```python
from build123d import *

# Parameters (mm, degrees)
F_9_64_0_14063_DIAMETER_HOLE2_D           = 3.572002
F_9_64_0_14063_DIAMETER_HOLE2_CSINK_D     = 4.842002
F_9_64_0_14063_DIAMETER_HOLE2_CSINK_ANGLE = 100
F_9_64_0_14063_DIAMETER_HOLE3_D           = 3.572002
F_9_64_0_14063_DIAMETER_HOLE3_CSINK_D     = 4.842002
F_9_64_0_14063_DIAMETER_HOLE3_CSINK_ANGLE = 100
CUT_EXTRUDE1_DEPTH                        = 3.81


with BuildPart() as part:
    # Sketch2 → Revolve1 (revolve)
    with BuildSketch(Plane.XY, mode=Mode.PRIVATE) as revolve1_sk:
        with BuildLine():
            Line((0, 0), (-35.56, 0))
            ThreePointArc((-35.56, 0), (-34.441376421, 45.516946226), (-48.26, 88.9))
            Line((-48.26, 88.9), (-50.8, 88.9))
            ThreePointArc((-50.8, 88.9), (-36.890578114, 45.529917412), (-38.1, 0))
            Line((-38.1, 0), (-38.1, -7.62))
            Line((-38.1, -7.62), (0, -7.62))
            Line((0, -7.62), (0, 0))
        make_face()
    revolve(revolve1_sk.sketch.rotate(Axis((0, 0, 0), (0, 1, 0)), 270), axis=Axis((0, 0, 0), (0, 1, 0)))

    # 9/64 (0.14063) Diameter Hole2 (through all)
    with Locations(Plane(origin=(0, 0, 0), x_dir=(1, 0, 0), z_dir=(0, 1, 0))):
        with Locations((0, -28.72641934), (-28.389650063, 0), (0, 28.72641934), (28.120234641, 0), (17.815094761, -20.105125845), (17.815094761, 19.431587291), (-18.421279459, 19.431587291), (-18.421279459, -20.105125845), (0, 0)):
            CounterSinkHole(F_9_64_0_14063_DIAMETER_HOLE2_D / 2, F_9_64_0_14063_DIAMETER_HOLE2_CSINK_D / 2, counter_sink_angle=F_9_64_0_14063_DIAMETER_HOLE2_CSINK_ANGLE)

    # 9/64 (0.14063) Diameter Hole3 (through all)
    with Locations(Plane(origin=(0, -7.62, 0), x_dir=(-1, 0, 0), z_dir=(0, -1, 0))):
        with Locations((-6.364939338, 18.960110303), (7.50995488, 18.960110303), (19.835710423, 7.914078013), (-19.29687958, 7.914078013), (-19.29687958, -8.385555001), (-7.038477892, -21.317495243), (7.914078013, -21.317495243), (19.835710423, -8.857031989)):
            CounterSinkHole(F_9_64_0_14063_DIAMETER_HOLE3_D / 2, F_9_64_0_14063_DIAMETER_HOLE3_CSINK_D / 2, counter_sink_angle=F_9_64_0_14063_DIAMETER_HOLE3_CSINK_ANGLE)

    # Sketch11 → Cut-Extrude1 (cut)
    with BuildSketch(Plane.XZ.offset(7.62)):
        with BuildLine():
            Line((-4.696611831, 37.809414665), (-4.696611831, 30.726938113))
            ThreePointArc((-4.696611831, 30.726938113), (-21.519829113, 22.429887281), (-30.506179441, 5.964554001))
            Line((-30.506179441, 5.964554001), (-37.630228482, 5.964554001))
            ThreePointArc((-37.630228482, 5.964554001), (-38.099253822, 0.238449554), (-37.701937681, -5.493077013))
            Line((-37.701937681, -5.493077013), (-30.594590918, -5.493077013))
            ThreePointArc((-30.594590918, -5.493077013), (-21.692260933, -22.263169229), (-4.696611831, -30.726938113))
            Line((-4.696611831, -30.726938113), (-4.696611831, -37.809414665))
            ThreePointArc((-4.696611831, -37.809414665), (0, -38.1), (4.696611831, -37.809414665))
            Line((4.696611831, -37.809414665), (4.696611831, -30.726938113))
            ThreePointArc((4.696611831, -30.726938113), (21.692260933, -22.263169229), (30.594590918, -5.493077013))
            Line((30.594590918, -5.493077013), (37.701937681, -5.493077013))
            ThreePointArc((37.701937681, -5.493077013), (38.099253822, 0.238449554), (37.630228482, 5.964554001))
            Line((37.630228482, 5.964554001), (30.506179441, 5.964554001))
            ThreePointArc((30.506179441, 5.964554001), (21.519829113, 22.429887281), (4.696611831, 30.726938113))
            Line((4.696611831, 30.726938113), (4.696611831, 37.809414665))
            ThreePointArc((4.696611831, 37.809414665), (0, 38.1), (-4.696611831, 37.809414665))
        make_face()
    extrude(amount=-CUT_EXTRUDE1_DEPTH, mode=Mode.SUBTRACT)


solid = part.part
```
Here's how the part is built. I have some questions about the finished solid (model axes, mm). A direction names the side the tool comes from. Round coordinates to 2 decimals unless told otherwise and drop trailing zeros. Loops run counter-clockwise (first coordinate to the right, second up) from the corner with the lowest first, then second, coordinate; pieces in that order, holes last.
1. Thinking about a two-plate mould opening in X: for faces 1 (the face through (0.387, -2.194, -26.983)), 2 (the face through (-34, -6, -5.493)), 3 (the face through (14.593, -3.863, -35.195)), which applies, released by +X, released by -X, zero draft, split by the parting line, or undercut?
Answers:
face 1: undercut
face 2: zero draft
face 3: split by the parting line
2. If I drill on probe 1 along Z at (x, y) = (5, 19); probe 2 along X at (y, z) = (57, 4); probe 3 along Z at (x, y) = (10.5, 61), over which ranges is the centre line in solid material (lowest first)?
Answers:
probe 1: z = -35.37 to -32.87, 32.87 to 35.37
probe 2: x = -38.83 to -36.36, 36.36 to 38.83
probe 3: z = -38.63 to -36.07, 36.07 to 38.63
3. Suppose I cut it at D-D, the plane y = 20.5. Please give me the cut outline in (x, z).
Answers:
outline: circle Ø71.3 at (0, 0); hole circle Ø66.35 at (0, 0)
4. Suppose I cut it at A-A, the plane x = 0. Please give me the cut outline in (y, z).
Answers:
outline: (-3.81, -38.1) - (0, -38.1) arc R135.83 cw to (88.9, -50.8) - (88.9, -48.26) arc R137.39 ccw to (0, -35.56) - (0, -31.15) - (-0.53, -30.51) - (-3.81, -30.51) - close; (-3.81, -26.94) - (-0.53, -26.94) - (0, -26.31) - (0, -2.42) - (-0.53, -1.79) - (-3.81, -1.79) - close; (-3.81, 1.79) - (-0.53, 1.79) - (0, 2.42) - (0, 26.31) - (-0.53, 26.94) - (-3.81, 26.94) - close; (-3.81, 30.51) - (-0.53, 30.51) - (0, 31.15) - (0, 35.56) arc R137.39 ccw to (88.9, 48.26) - (88.9, 50.8) arc R135.83 cw to (0, 38.1) - (-3.81, 38.1) - close
5. Suppose I cut it at C-C, the plane y = 81. Please give me the cut outline in (x, z).
Answers:
outline: circle Ø94.03 at (0, 0); hole circle Ø89.02 at (0, 0)
6. For faces 4 (the face through (4.697, -6, 34)), 5 (the face through (19, 88.9, 45)), 6 (the face through (8, -3.81, 1)), which set-ups out of +Z, -Z, +X, -X, +Y, -Y let a thin tool reach every point of the face, with its end or its side?
Answers:
face 4: +Z, -Z, -Y
face 5: +Z, -Z, +X, -X, +Y
face 6: -Y
7. Will these pins go through, and if not, where does the flat tip stop? pin 1 (3 mm diameter, centred on x = 34.5, y = -6, fed in from -Z); pin 2 (4 mm diameter, centred on x = -18.42, z = 20.11, fed in from -Y); pin 3 (4 mm diameter, centred on y = 77, z = 10, fed in from -X); pin 4 (2 mm diameter, centred on x = 0, z = 0, fed in from -Y).
Answers:
pin 1: stops at z = -19.04
pin 2: stops at y = -3.81
pin 3: stops at x = -45.16
pin 4: passes through
8. Suppose I cut it at B-B, the plane z = 0. Please give me the cut outline in (x, y), and give its area (3 significant figures).
Answers:
outline: (-50.8, 88.9) arc R135.83 cw to (-38.1, 0) - (-38.1, -3.81) - (-30.18, -3.81) - (-30.18, -0.53) - (-30.81, 0) - (-35.56, 0) arc R137.39 ccw to (-48.26, 88.9) - close; (-26.6, -3.81) - (-1.79, -3.81) - (-1.79, -0.53) - (-2.42, 0) - (-25.97, 0) - (-26.6, -0.53) - close; (1.79, -3.81) - (26.33, -3.81) - (26.33, -0.53) - (25.7, 0) - (2.42, 0) - (1.79, -0.53) - close; (29.91, -3.81) - (38.1, -3.81) - (38.1, 0) arc R135.83 cw to (50.8, 88.9) - (48.26, 88.9) arc R137.39 ccw to (35.56, 0) - (30.54, 0) - (29.91, -0.53) - close
area: 689 mm2
